Part model, mm, in its own coordinate system. A direction names the side the tool comes from. Give positions to 0.01 mm unless a question says otherwise; leave off trailing zeros. Order: outer loops, then holes, each group sorted by start corner. A loop starts at its lowest first (then second) coordinate and runs counter-clockwise, first axis right, second up. Notation, with made-up numbers: (6.5, 83.5) - (32.5, 83.5) arc R16 ccw to (32.5, 101.5) - close; hole circle Ø9 at (15, 83.25). An arc over 180 degrees is marked (long way). Use one line per item in the form item = value. Start each with the question number.
1. Tool access for faces 5 (the face through (52.84, -1.479, 17.816)), 6 (the face through (20, -3, 3)), 7 (the face through (-11.921, -1, -3)): list every direction of +Z, -Z, +X, -X, +Y, -Y with a clear straight run to the whole face (end or side of a thin tool).
2. Band-saw the part on D-D, the plane x = 3. List the corners of the cut face in (y, z), plus the area to 3 significant figures.
3. Band-saw the part on A-A, the plane x = 14. List the corners of the cut face in (y, z).
4. Pin check, flat tips, straight feed: P1, Ø12, axis at x = 43, z = -7.5, coming from the -Y side; P2, Ø1.8, axis at x = 5, y = -1, coming from the +Z side; P3, Ø0.8, axis at x = -10, y = -1, coming from the -Z side; P4, Ø0.8, axis at x = -10.5, y = -2, coming from the -Z side. Stop position of each tip, or through.
5. Drill centre lines: line 1 (X direction, y = -2.45, z = 6.5); line 2 (Z direction, x = 23.5, y = -1.85); line 3 (X direction, y = -2.1, z = 8). Where is each one in solid material? Low to high.
6. Band-saw the part on B-B, the plane z = 6.5. State how many separate pieces and enclosed holes the cut face has, plus the area to 3 significant figures.
7. Pull direction Z, two halves, no side cores. Call faces 1 (the face through (40.94, -1.48, -7.97)), 2 (the face through (20, 0, 3)), 3 (the face through (15, -1, 13.67)), 4 (the face through (-9.184, -1, 3)): +Z half, -Z half, draft (parallel to the pull), parting line (faces both ways), or undercut.
from build123d import *

# Parameters (mm, degrees)
F0_W     = 2.7374038473
F0_H     = 4.5464726281
F1_DEPTH = 3


with BuildPart() as f1:
    # F0 (on Front) → F1 (new body)
    with BuildSketch(Plane.XZ):
        with BuildLine():
            Line((-13.9879264009, 8.4983842463), (-10.7078288449, 8.4983842463))
            ThreePointArc((-10.7078288449, 8.4983842463), (-12.3096819162, -5.9457433928), (0, -13.6704108706))
            Line((0, -13.6704108706), (29.832560569, -13.6704108706))
            ThreePointArc((29.832560569, -13.6704108706), (41.0439649972, -7.8220549805), (42.6626390029, 4.7190275219))
            ThreePointArc((42.6626390029, 4.7190275219), (52.7277631814, 0.6811115523), (57.2114773095, -9.193492122))
            Line((57.2114773095, -9.193492122), (57.2114773095, 27.5829305145))
            ThreePointArc((57.2114773095, 27.5829305145), (52.7277631814, 17.7083268402), (42.6626390029, 13.6704108706))
            Line((42.6626390029, 13.6704108706), (29.832560569, 13.6704108706))
            Line((29.832560569, 13.6704108706), (0, 13.6704108706))
            Line((0, 13.6704108706), (-14.4307379611, 13.6704108706))
            Line((-14.4307379611, 13.6704108706), (-14.8297163701, 14.5122008398))
            Line((-14.8297163701, 14.5122008398), (-15.268201828, 14.5122008398))
            ThreePointArc((-15.268201828, 14.5122008398), (-15.9753086092, 14.219307621), (-16.268201828, 13.5122008398))
            Line((-16.268201828, 13.5122008398), (-16.268201828, 9.0994058373))
            ThreePointArc((-16.268201828, 9.0994058373), (-15.9753086092, 8.3922990562), (-15.268201828, 8.0994058373))
            Line((-15.268201828, 8.0994058373), (-14.8297163701, 8.0994058373))
            Line((-14.8297163701, 8.0994058373), (-13.9879264009, 8.4983842463))
        make_face()
        with Locations((-10.5523099191, -3.12910098)):
            Rectangle(F0_W, F0_H, mode=Mode.SUBTRACT)
        with BuildLine():
            add(Edge.make_bspline(
                [(0.173976751, -10.791644976), (-1.0682128711, -12.1435613479), (-3.3993887284, -12.1435613479)],
                knots=[0, 0, 0, 1, 1, 1], degree=2))
            add(Edge.make_bspline(
                [(-3.3993887284, -12.1435613479), (-4.6125939259, -12.1435613479), (-5.3123607464, -11.7957482538)],
                knots=[0, 0, 0, 1, 1, 1], degree=2))
            Line((-5.3123607464, -11.7957482538), (-5.3123607464, -9.9200419245))
            add(Edge.make_bspline(
                [(-5.3123607464, -9.9200419245), (-4.393140426, -10.176761113), (-3.3993887284, -10.176761113)],
                knots=[0, 0, 0, 1, 1, 1], degree=2))
            add(Edge.make_bspline(
                [(-3.3993887284, -10.176761113), (-2.1157927856, -10.176761113), (-1.4491510218, -9.4003925993)],
                knots=[0, 0, 0, 1, 1, 1], degree=2))
            add(Edge.make_bspline(
                [(-1.4491510218, -9.4003925993), (-0.782509258, -8.6240240855), (-0.782509258, -7.1623809636)],
                knots=[0, 0, 0, 1, 1, 1], degree=2))
            Line((-0.782509258, -7.1623809636), (-0.782509258, 11.7561669801))
            Line((-0.782509258, 11.7561669801), (1.416166373, 11.7561669801))
            Line((1.416166373, 11.7561669801), (1.416166373, -6.9801931523))
            add(Edge.make_bspline(
                [(1.416166373, -6.9801931523), (1.416166373, -9.439728604), (0.173976751, -10.791644976)],
                knots=[0, 0, 0, 1, 1, 1], degree=2))
        make_face(mode=Mode.SUBTRACT)
        with Locations((-10.5523099191, 3.0826488801)):
            Rectangle(F0_W, F0_H, mode=Mode.SUBTRACT)
        Polygon((20.6038554014, -7.1623809636), (18.326507761, -7.1623809636), (15.9704881112, -1.1460425608), (8.3889907847, -1.1460425608), (6.0619555594, -7.1623809636), (3.8342955039, -7.1623809636), (11.3122770286, 11.8348389895), (13.1631395654, 11.8348389895), align=None, mode=Mode.SUBTRACT)
        with BuildLine():
            add(Edge.make_bspline(
                [(32.7607511691, 1.0277892777), (33.8787218289, -0.1895565519), (33.8787218289, -2.1273723622)],
                knots=[0, 0, 0, 1, 1, 1], degree=2))
            add(Edge.make_bspline(
                [(33.8787218289, -2.1273723622), (33.8787218289, -4.6241735025), (32.0671952968, -6.0237071434)],
                knots=[0, 0, 0, 1, 1, 1], degree=2))
            add(Edge.make_bspline(
                [(32.0671952968, -6.0237071434), (30.2556687647, -7.4232407842), (27.1501947096, -7.4232407842)],
                knots=[0, 0, 0, 1, 1, 1], degree=2))
            add(Edge.make_bspline(
                [(27.1501947096, -7.4232407842), (23.7880014659, -7.4232407842), (21.9744046177, -6.5537080488)],
                knots=[0, 0, 0, 1, 1, 1], degree=2))
            Line((21.9744046177, -6.5537080488), (21.9744046177, -4.4337044272))
            add(Edge.make_bspline(
                [(21.9744046177, -4.4337044272), (23.1420628625, -4.9222990118), (24.5126120788, -5.2080026249)],
                knots=[0, 0, 0, 1, 1, 1], degree=2))
            add(Edge.make_bspline(
                [(24.5126120788, -5.2080026249), (25.8831612951, -5.493706238), (27.228866719, -5.493706238)],
                knots=[0, 0, 0, 1, 1, 1], degree=2))
            add(Edge.make_bspline(
                [(27.228866719, -5.493706238), (29.42754235, -5.493706238), (30.5413723777, -4.6593688752)],
                knots=[0, 0, 0, 1, 1, 1], degree=2))
            add(Edge.make_bspline(
                [(30.5413723777, -4.6593688752), (31.6552024055, -3.8250315124), (31.6552024055, -2.3344039659)],
                knots=[0, 0, 0, 1, 1, 1], degree=2))
            add(Edge.make_bspline(
                [(31.6552024055, -2.3344039659), (31.6552024055, -1.3530741645), (31.2597720425, -0.7257684054)],
                knots=[0, 0, 0, 1, 1, 1], degree=2))
            add(Edge.make_bspline(
                [(31.2597720425, -0.7257684054), (30.8643416795, -0.0984626462), (29.938910411, 0.4336085752)],
                knots=[0, 0, 0, 1, 1, 1], degree=2))
            add(Edge.make_bspline(
                [(29.938910411, 0.4336085752), (29.0134791426, 0.9656797966), (27.1253509171, 1.6364621925)],
                knots=[0, 0, 0, 1, 1, 1], degree=2))
            add(Edge.make_bspline(
                [(27.1253509171, 1.6364621925), (24.4877682863, 2.5805263053), (23.3553054142, 3.8744738282)],
                knots=[0, 0, 0, 1, 1, 1], degree=2))
            add(Edge.make_bspline(
                [(23.3553054142, 3.8744738282), (22.2228425422, 5.1684213512), (22.2228425422, 7.2511592841)],
                knots=[0, 0, 0, 1, 1, 1], degree=2))
            add(Edge.make_bspline(
                [(22.2228425422, 7.2511592841), (22.2228425422, 9.4374130189), (23.8646031593, 10.7313605419)],
                knots=[0, 0, 0, 1, 1, 1], degree=2))
            add(Edge.make_bspline(
                [(23.8646031593, 10.7313605419), (25.5063637764, 12.0253080648), (28.2143371524, 12.0253080648)],
                knots=[0, 0, 0, 1, 1, 1], degree=2))
            add(Edge.make_bspline(
                [(28.2143371524, 12.0253080648), (31.0341075945, 12.0253080648), (33.4025491405, 10.9901500465)],
                knots=[0, 0, 0, 1, 1, 1], degree=2))
            Line((33.4025491405, 10.9901500465), (32.7152042163, 9.0771780285))
            add(Edge.make_bspline(
                [(32.7152042163, 9.0771780285), (30.3716064627, 10.05850783), (28.1605089355, 10.05850783)],
                knots=[0, 0, 0, 1, 1, 1], degree=2))
            add(Edge.make_bspline(
                [(28.1605089355, 10.05850783), (26.4131622005, 10.05850783), (25.429762083, 9.3090534247)],
                knots=[0, 0, 0, 1, 1, 1], degree=2))
            add(Edge.make_bspline(
                [(25.429762083, 9.3090534247), (24.4463619656, 8.5595990194), (24.4463619656, 7.2263154917)],
                knots=[0, 0, 0, 1, 1, 1], degree=2))
            add(Edge.make_bspline(
                [(24.4463619656, 7.2263154917), (24.4463619656, 6.2449856903), (24.808667272, 5.6156096151)],
                knots=[0, 0, 0, 1, 1, 1], degree=2))
            add(Edge.make_bspline(
                [(24.808667272, 5.6156096151), (25.1709725785, 4.98623354), (26.0322240497, 4.4624435827)],
                knots=[0, 0, 0, 1, 1, 1], degree=2))
            add(Edge.make_bspline(
                [(26.0322240497, 4.4624435827), (26.893475521, 3.9386536254), (28.6656660485, 3.3051369181)],
                knots=[0, 0, 0, 1, 1, 1], degree=2))
            add(Edge.make_bspline(
                [(28.6656660485, 3.3051369181), (31.6427805093, 2.2451351073), (32.7607511691, 1.0277892777)],
                knots=[0, 0, 0, 1, 1, 1], degree=2))
        make_face(mode=Mode.SUBTRACT)
    extrude(amount=F1_DEPTH)


solid = f1.part
From the geometry:
q1.face_5 = +Z, +Y, -Y
q1.face_6 = +Z, -Z, +X, -X, -Y
q1.face_7 = +Y, -Y
q2.outline = (-3, -13.67) - (0, -13.67) - (0, 13.67) - (-3, 13.67) - close
q2.area = 82.0 mm²
q3.outline = (-3, -13.67) - (0, -13.67) - (0, -1.15) - (-3, -1.15) - close; (-3, 9.7) - (0, 9.7) - (0, 13.67) - (-3, 13.67) - close
q4.P1 = -3
q4.P2 = 13.67
q4.P3 = -9.73
q4.P4 = -9.21
q5.line_1 = -12.03 to -0.78, 1.42 to 9.21, 15.25 to 22.26, 24.5 to 57.21
q5.line_2 = -13.67 to -7.07, -4.96 to 3.72, 10.41 to 13.67
q5.line_3 = -11.09 to -0.78, 1.42 to 9.8, 14.67 to 22.27, 24.54 to 57.21
q6.separate_pieces = 4
q6.enclosed_holes = 0
q6.area = 176 mm²
q7.face_1 = undercut
q7.face_2 = draft
q7.face_3 = +Z half
q7.face_4 = undercut
